Check sheet for the modelled part. Datum: model origin and axes. Units: mm. Face numbers are marked on the shaded views. Give positions to 0.01 mm unless a question says otherwise; leave off trailing zeros. Loops run counter-clockwise (first coordinate to the right, second up) from the corner with the lowest first, then second, coordinate; pieces in that order, holes last. Notation, with made-up numbers: M 45.5,2.25 L 64.5,2.25 A21 ccw 64.5,27.25 Z; hole C 36.25,-17.5 d9. An arc over 180 degrees is marked long. Write each question's results on one line, items separated by ' | '. Start each with the question number.
1. Sectioned sample at D-D on x = -50. Record the cut outline in (y, z), and give its area (3 significant figures).
2. Sectioned sample at A-A on x = 0. Give the number of separate pieces and of enclosed holes in the cut face, and give its area (3 significant figures).
3. Go/stop test with flat-tipped pins: pin 1 (5 mm diameter, centred on x = 25, z = -17.5, fed in from +Y); pin 2 (1.5 mm diameter, centred on x = 31.5, y = -2.5, fed in from -Z); pin 3 (4.5 mm diameter, centred on x = 50, z = 0, fed in from -Y). Record where each tip stops, or that it passes through.
4. Sectioned sample at B-B on z = 50. Record the cut outline in (x, y).
5. Material ranges on line 1 along Z through (x, y) = (-36.5, -3.5); line 2 along X through (y, z) = (0.25, -34); line 3 along Z through (x, y) = (38.5, -3.5), recorded low to high.
6. Draft check along X on the marked faces 1 and 2. Enter one of: pulls with the +X half, pulls with the -X half, needs draft (parallel to the pull), parting line crosses it, or undercut.
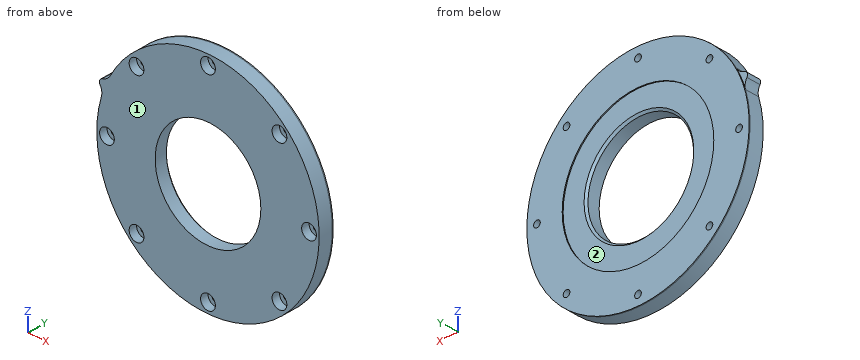
```python
from build123d import *

# Parameters (mm, degrees)
SKETCH1_R           = 55
SKETCH1_R_2         = 37.5
SKETCH1_R_3         = 1.65
BOSS_EXTRUDE1_DEPTH = 0.5
SKETCH2_R           = 26.15
SKETCH2_R_2         = 1.65
BOSS_EXTRUDE2_DEPTH = 7
CHAMFER1_SIZE       = 1
SKETCH3_R           = 3.65
SKETCH3_R_2         = 1.65
CUT_EXTRUDE1_DEPTH  = 4


with BuildPart() as part:
    # Sketch1 → Boss-Extrude1 (new body)
    with BuildSketch(Plane(origin=(0, 0, 0), x_dir=(1, 0, 0), z_dir=(0, 1, 0))):
        Circle(SKETCH1_R)
        Circle(SKETCH1_R_2, mode=Mode.SUBTRACT)
        with Locations((0, 50)):
            Circle(SKETCH1_R_3, mode=Mode.SUBTRACT)
        with Locations((35.355339059, 35.355339059)):
            Circle(SKETCH1_R_3, mode=Mode.SUBTRACT)
        with Locations((50, 0)):
            Circle(SKETCH1_R_3, mode=Mode.SUBTRACT)
        with Locations((35.355339059, -35.355339059)):
            Circle(SKETCH1_R_3, mode=Mode.SUBTRACT)
        with Locations((0, -50)):
            Circle(SKETCH1_R_3, mode=Mode.SUBTRACT)
        with Locations((-35.355339059, -35.355339059)):
            Circle(SKETCH1_R_3, mode=Mode.SUBTRACT)
        with Locations((-50, 0)):
            Circle(SKETCH1_R_3, mode=Mode.SUBTRACT)
        with Locations((-35.355339059, 35.355339059)):
            Circle(SKETCH1_R_3, mode=Mode.SUBTRACT)
    extrude(amount=BOSS_EXTRUDE1_DEPTH)

    # Sketch2 → Boss-Extrude2 (add)
    with BuildSketch(Plane.XZ):
        with BuildLine():
            ThreePointArc((-52.76902678, 15.505799326), (50.813374288, -21.04758878), (-48.277592523, 26.349080822))
            ThreePointArc((-48.277592523, 26.349080822), (-49.915423513, 24.445273361), (-52.189000111, 23.37858566))
            ThreePointArc((-52.189000111, 23.37858566), (-53.585012886, 22.195639077), (-53.434352336, 20.372039427))
            ThreePointArc((-53.434352336, 20.372039427), (-52.580953013, 18.01011589), (-52.76902678, 15.505799326))
        make_face()
        Circle(SKETCH2_R, mode=Mode.SUBTRACT)
        with Locations((0, -50)):
            Circle(SKETCH2_R_2, mode=Mode.SUBTRACT)
        with Locations((35.355339059, -35.355339059)):
            Circle(SKETCH2_R_2, mode=Mode.SUBTRACT)
        with Locations((50, 0)):
            Circle(SKETCH2_R_2, mode=Mode.SUBTRACT)
        with Locations((35.355339059, 35.355339059)):
            Circle(SKETCH2_R_2, mode=Mode.SUBTRACT)
        with Locations((0, 50)):
            Circle(SKETCH2_R_2, mode=Mode.SUBTRACT)
        with Locations((-35.355339059, 35.355339059)):
            Circle(SKETCH2_R_2, mode=Mode.SUBTRACT)
        with Locations((-50, 0)):
            Circle(SKETCH2_R_2, mode=Mode.SUBTRACT)
        with Locations((-35.355339059, -35.355339059)):
            Circle(SKETCH2_R_2, mode=Mode.SUBTRACT)
    extrude(amount=BOSS_EXTRUDE2_DEPTH)

    # Chamfer1
    chamfer1_edges = [part.edges().sort_by_distance(p)[0] for p in [
        (-26.15, 0, 0),
    ]]
    chamfer(chamfer1_edges, length=CHAMFER1_SIZE)

    # Sketch3 → Cut-Extrude1 (cut)
    with BuildSketch(Plane.XZ.offset(7)):
        with Locations((-50, 0)):
            Circle(SKETCH3_R)
        with Locations((-50, 0)):
            Circle(SKETCH3_R_2, mode=Mode.SUBTRACT)
        with Locations((-35.355339059, -35.355339059)):
            Circle(SKETCH3_R)
        with Locations((-35.355339059, -35.355339059)):
            Circle(SKETCH3_R_2, mode=Mode.SUBTRACT)
        with Locations((0, -50)):
            Circle(SKETCH3_R)
        with Locations((0, -50)):
            Circle(SKETCH3_R_2, mode=Mode.SUBTRACT)
        with Locations((35.355339059, -35.355339059)):
            Circle(SKETCH3_R)
        with Locations((35.355339059, -35.355339059)):
            Circle(SKETCH3_R_2, mode=Mode.SUBTRACT)
        with Locations((50, 0)):
            Circle(SKETCH3_R)
        with Locations((50, 0)):
            Circle(SKETCH3_R_2, mode=Mode.SUBTRACT)
        with Locations((35.355339059, 35.355339059)):
            Circle(SKETCH3_R)
        with Locations((35.355339059, 35.355339059)):
            Circle(SKETCH3_R_2, mode=Mode.SUBTRACT)
        with Locations((0, 50)):
            Circle(SKETCH3_R)
        with Locations((0, 50)):
            Circle(SKETCH3_R_2, mode=Mode.SUBTRACT)
        with Locations((-35.355339059, 35.355339059)):
            Circle(SKETCH3_R)
        with Locations((-35.355339059, 35.355339059)):
            Circle(SKETCH3_R_2, mode=Mode.SUBTRACT)
    extrude(amount=-CUT_EXTRUDE1_DEPTH, mode=Mode.SUBTRACT)


solid = part.part
```
Output values:
1) outline: M -7,-22.91 L 0.5,-22.91 L 0.5,-1.65 L -3,-1.65 L -3,-3.65 L -7,-3.65 Z; M -7,3.65 L -3,3.65 L -3,1.65 L 0.5,1.65 L 0.5,22.91 L 0,22.91 L 0,24.38 L -7,24.38 Z | area: 313 mm2
2) separate pieces: 4 | enclosed holes: 0 | area: 339 mm2
3) pin 1: y = 0 | pin 2: z = -45.6 | pin 3: y = -3
4) outline: M -22.91,-7 L -3.65,-7 L -3.65,-3 L -1.65,-3 L -1.65,0.5 L -22.91,0.5 Z; M 1.65,-3 L 3.65,-3 L 3.65,-7 L 22.91,-7 L 22.91,0.5 L 1.65,0.5 Z
5) line 1: -41.14 to -38.82, -31.89 to 31.89, 38.82 to 41.14 | line 2: -43.23 to -36.3, -34.41 to -15.82, 15.82 to 34.41, 36.3 to 43.23 | line 3: -39.28 to -37.21, -33.5 to 33.5, 37.21 to 39.28
6) face 1: needs draft | face 2: undercut
